Could you check a few things on this model? Use its own coordinates, in mm. A direction names the side the tool comes from. Give positions to 0.01 mm unless a question says otherwise; leave off trailing zeros. Write each loop counter-clockwise with the first axis right and the second up, starting at its lowest first coordinate (ties: lowest second). Pieces come first, ordered by that corner, then holes. Notation, with made-up numbers: M -28,49.25 L 7,49.25 A21 ccw 7,63.25 Z; hole C -24.75,-15.5 d4. An arc over 180 degrees is marked long. Answer as a JSON object with one key per item and string values. Group by question number.
```python
from build123d import *

# Parameters (mm, degrees)
EXTRUDE_1_DEPTH     = 9
SKETCH_2_R          = 2.55
CUT_EXTRUDE_1_DEPTH = 106.190303736
SKETCH_3_R          = 2.55
CUT_EXTRUDE_2_DEPTH = 106.190303736


with BuildPart() as part:
    # 草图1 → 凸台-拉伸1 (new, symmetric)
    with BuildSketch(Plane.XY):
        Polygon((0, 78), (0, 0), (-78, 0), (-78, 8), (-8, 8), (-8, 78), align=None)
    extrude(amount=EXTRUDE_1_DEPTH, both=True)

    # 草图2 → 切除-拉伸1 (cut, through all)
    with BuildSketch(Plane(origin=(0, 8, 0), x_dir=(1, 0, 0), z_dir=(0, 1, 0))):
        with Locations(Location((-68, 0, 0), (0, 0, 180))):
            Circle(SKETCH_2_R)
        with Locations(Location((-40, 0, 0), (0, 0, 180))):
            Circle(SKETCH_2_R)
    extrude(amount=-CUT_EXTRUDE_1_DEPTH, mode=Mode.SUBTRACT)

    # 草图3 → 切除-拉伸2 (cut, through all)
    with BuildSketch(Plane.ZY.offset(8)):
        with Locations(Location((0, 40, 0), (0, 0, 270))):
            Circle(SKETCH_3_R)
        with Locations(Location((0, 68, 0), (0, 0, 270))):
            Circle(SKETCH_3_R)
    extrude(amount=-CUT_EXTRUDE_2_DEPTH, mode=Mode.SUBTRACT)


solid = part.part
```
1) I'm going to push flat-ended pins straight in: pin 1 (6 mm diameter, centred on y = 68, z = 0, fed in from -X); pin 2 (8 mm diameter, centred on x = -40, z = 0, fed in from +Y). Where does each tip first touch, or does it pass through?
2) If we section it at B-B, the plane y = 6.5: List the corners of the cut face in (x, z) for me.
3) Please list where these lines run through material, in increasing order: line 1 along Z through (x, y) = (-40, 4.5); line 2 along X through (y, z) = (4, -0.25); line 3 along X through (y, z) = (32, 2.5). Write a range as from..to.
4) We'd pull the mould along Z, two halves only. Please class faces 3 (the flat face through (-78, 4, 0)), 4 (the cylindrical face through (-37.452, 4.056, 0.112)), 5 (the flat face through (-21, 7, 9)), 6 (the cylindrical face through (-4.056, 70.548, 0.112)): released by +Z, released by -Z, zero draft, split by the parting line, or undercut.
5) For faces 1 (the flat face through (-8, 43, 2)), 2 (the flat face through (-4, 78, 0)), which set-ups out of +Z, -Z, +X, -X, +Y, -Y let a thin tool reach every point of the face, with its end or its side?
6) If we section it at D-D, the plane z = -1: List the corners of the cut face in (x, y) for me.
7) If we section it at A-A, the plane x = -68: List the corners of the cut face in (y, z) for me.
8) If we section it at C-C, the plane y = 40: List the corners of the cut face in (x, z) for me, plus the area to 3 significant figures.
Taken from the geometry:
{
 "1": {"pin 1": "x = -8", "pin 2": "y = 8"},
 "2": {"outline": "M -78,-9 L 0,-9 L 0,9 L -78,9 Z; hole C -68,0 d5.1; hole C -40,0 d5.1"},
 "3": {"line 1": "-9..-2.55, 2.55..9", "line 2": "-78..-70.54, -65.46..-42.54, -37.46..0", "line 3": "-8..0"},
 "4": {"face 3": "zero draft", "face 4": "undercut", "face 5": "released by +Z", "face 6": "undercut"},
 "5": {"face 1": "+Z, -Z, -X, +Y", "face 2": "+Z, -Z, +X, -X, +Y"},
 "6": {"outline": "M -78,0 L -70.35,0 L -70.35,8 L -78,8 Z; M -65.65,0 L -42.35,0 L -42.35,8 L -65.65,8 Z; M -37.65,0 L 0,0 L 0,37.65 L -8,37.65 L -8,8 L -37.65,8 Z; M -8,42.35 L 0,42.35 L 0,65.65 L -8,65.65 Z; M -8,70.35 L 0,70.35 L 0,78 L -8,78 Z"},
 "7": {"outline": "M 0,-9 L 8,-9 L 8,-2.55 L 0,-2.55 Z; M 0,2.55 L 8,2.55 L 8,9 L 0,9 Z"},
 "8": {"outline": "M -8,-9 L 0,-9 L 0,-2.55 L -8,-2.55 Z; M -8,2.55 L 0,2.55 L 0,9 L -8,9 Z", "area": "103 mm²"}
}
